Can you work these out from the model? Positions are in its coordinate system, mm. A direction names the side the tool comes from. Give positions to 0.01 mm unless a question says otherwise; leave off trailing zeros. Write each loop counter-clockwise with the first axis right and the second up, starting at its lowest first coordinate (ties: lowest second). Pieces come first, ordered by that corner, then holes.
from build123d import *

# Parameters (mm, degrees)
F0_R     = 1.15
F1_DEPTH = 2
F2_R     = 1.5
F3_DEPTH = 5
F4_R     = 1.49999


# Not quite as in the source:
# - a fillet or chamfer is up to 0.001 mm smaller than in the source, because OpenCascade refuses the exact size


with BuildPart() as f1:
    # F0 (on Right) → F1 (new body, symmetric)
    with BuildSketch(Plane.YZ):
        with BuildLine():
            Line((5, -3.1), (5, 3.1))
            Line((5, 3.1), (-3.5, 3.1))
            ThreePointArc((-3.5, 3.1), (-3.9393398282, 2.0393398282), (-5, 1.6))
            Line((-5, 1.6), (-5, -1.6))
            ThreePointArc((-5, -1.6), (-3.9393398282, -2.0393398282), (-3.5, -3.1))
            Line((-3.5, -3.1), (5, -3.1))
        make_face()
        with Locations((2.5, 0)):
            Circle(F0_R, mode=Mode.SUBTRACT)
    extrude(amount=F1_DEPTH, both=True)

    # F2 (on face) → F3 (cut)
    with BuildSketch(Plane.XZ.offset(5)):
        Circle(F2_R)
    extrude(amount=-F3_DEPTH, mode=Mode.SUBTRACT)

    # F4 (radius 1.5 in the source; OpenCascade refuses exactly that, so slightly less here)
    f4_edges = [f1.edges().sort_by_distance(p)[0] for p in [
        (0, -3.5, 3.1),
        (0, -3.5, -3.1),
        (2, 0.75, -3.1),
        (2, 0.75, 3.1),
        (0, 5, 3.1),
        (0, 5, -3.1),
        (-2, 0.75, 3.1),
        (-2, 0.75, -3.1),
    ]]
    fillet(f4_edges, radius=F4_R)


solid = f1.part
(1) If we mould it in two halves opening along X, with no side actions, what happens to faces 1 (the face through (-0.028, 3.562, -0.44)), 2 (the face through (0, 0, 0)), 3 (the face through (-1.57, 0.07, -2.65)), 4 (the face through (1.55, -0.07, 2.67))? For each: +X half, -X half, draft (parallel to the pull), parting line (faces both ways), or undercut.
Returned:
face 1: draft
face 2: undercut
face 3: -X half
face 4: +X half
(2) Imagine slicing it at C-C, the plane x = 0. Write out the boundary of the cut face in (y, z), plus the area to 3 significant figures.
Returned:
outline: (-5, -1.6) arc R1.5 cw to (-3.7, -2.35) arc R1.5 ccw to (-2.4, -3.1) - (3.5, -3.1) arc R1.5 ccw to (5, -1.6) - (5, 1.6) arc R1.5 ccw to (3.5, 3.1) - (-2.4, 3.1) arc R1.5 ccw to (-3.7, 2.35) arc R1.5 cw to (-5, 1.6) - (-5, 1.5) - (0, 1.5) - (0, -1.5) - (-5, -1.5) - close; hole circle Ø2.3 at (2.5, 0)
area: 38.0 mm2
(3) If I drill on L1, parallel to Z at x = 0.3, y = 2.5; L2, parallel to Z at x = 0, y = -1.95; L3, parallel to Y at x = -0.65, z = 0.25, over which ranges is the centre line in solid material (lowest first)?
Returned:
L1: z = -3.1 to -1.15, 1.15 to 3.1
L2: z = -3.1 to -1.5, 1.5 to 3.1
L3: y = 0 to 1.38, 3.62 to 5
(4) Imagine slicing it at B-B, the plane y = 2.5. Write out the boundary of the cut face in (x, z), plus the area to 3 significant figures.
Returned:
outline: (-2, -1.6) arc R1.5 ccw to (-0.5, -3.1) - (0.5, -3.1) arc R1.5 ccw to (2, -1.6) - (2, -1.15) - (-2, -1.15) - close; (-2, 1.15) - (2, 1.15) - (2, 1.6) arc R1.5 ccw to (0.5, 3.1) - (-0.5, 3.1) arc R1.5 ccw to (-2, 1.6) - close
area: 13.7 mm2
(5) For faces 5 (the face through (-1.5, -2.54, 0.07)), 6 (the face through (0.9, -5, 1.4)), which set-ups out of +Z, -Z, +X, -X, +Y, -Y let a thin tool reach every point of the face, with its end or its side?
Returned:
face 5: -Y
face 6: +Z, -Z, +X, -X, -Y
(6) Imagine slicing it at A-A, the plane z = 0. Write out the boundary of the cut face in (x, y).
Returned:
outline: (-2, -5) - (-1.5, -5) - (-1.5, 0) - (1.5, 0) - (1.5, -5) - (2, -5) - (2, 1.35) - (-2, 1.35) - close; (-2, 3.65) - (2, 3.65) - (2, 5) - (-2, 5) - close
(7) Imagine slicing it at D-D, the plane y = 0.75. Write out the boundary of the cut face in (x, z), plus the area to 3 significant figures.
Returned:
outline: (-2, -1.6) arc R1.5 ccw to (-0.5, -3.1) - (0.5, -3.1) arc R1.5 ccw to (2, -1.6) - (2, 1.6) arc R1.5 ccw to (0.5, 3.1) - (-0.5, 3.1) arc R1.5 ccw to (-2, 1.6) - close
area: 22.9 mm2
(8) Will this pin go through, and if not, where does the flat tip stop? P1, Ø1.5, axis at x = 0, y = -3.5, coming from the -Z side.
Returned:
P1: stops at z = -3.06
